Check sheet for the drawn part. Datum: minimum x, y, z corner. Units: mm. A direction names the side the tool comes from. Coordinates: 2 decimals unless noted, no trailing zeros. Order: outer loops, then holes, each group sorted by start corner. A loop starts at its lowest first (then second) coordinate and runs counter-clockwise, first axis right, second up.
Q1. Cross-section at C-C, the plane x = 6. Record the boundary of the cut face in (y, z).
Q2. Cross-section at B-B, the plane z = 5. Record the boundary of the cut face in (x, y), and give its area (3 significant figures).
Q3. Draft check along Z on the marked faces 5, 6, 7 and 8. Enter one of: pulls with the +Z half, pulls with the -Z half, needs draft (parallel to the pull), parting line crosses it, or undercut.
Q4. Thickness scan on line 1 (Y direction, x = 15, z = 45); line 2 (X direction, y = 14, z = 36); line 3 (Z direction, x = 28.5, y = 9.5). Record the ranges inside material, lowest first.
Q5. Set-up check for the marked faces 1, 2, 3 and 4: record each of +Z, -Z, +X, -X, +Y, -Y from which the full face is reachable in a straight line by a thin tool's end or side.
Q6. Depth check by flat-ended pin: P1, Ø1.6, axis at x = 51, y = 1.5, coming from the +Z side; P2, Ø1, axis at x = 47, z = 16.5, coming from the +Y side; P3, Ø1, axis at x = 40.5, y = 1, coming from the -Z side. Enter the tip coordinate at first touch or a pass-through.
Q7. Cross-section at A-A, the plane y = 9.75. Record the boundary of the cut face in (x, z), and give its area (3 significant figures).
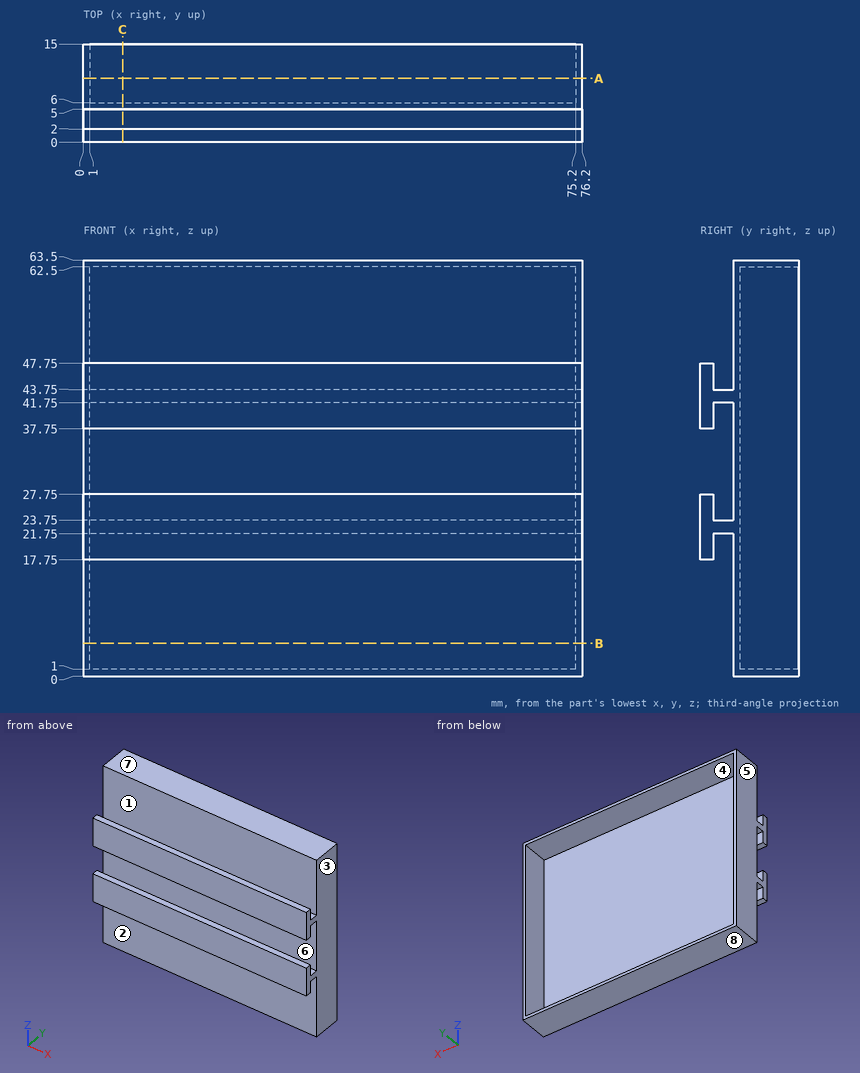
Check values:
1. outline: (0, 17.75) - (2, 17.75) - (2, 21.75) - (5, 21.75) - (5, 0) - (15, 0) - (15, 1) - (6, 1) - (6, 62.5) - (15, 62.5) - (15, 63.5) - (5, 63.5) - (5, 43.75) - (2, 43.75) - (2, 47.75) - (0, 47.75) - (0, 37.75) - (2, 37.75) - (2, 41.75) - (5, 41.75) - (5, 23.75) - (2, 23.75) - (2, 27.75) - (0, 27.75) - close
2. outline: (0, 5) - (76.2, 5) - (76.2, 15) - (75.2, 15) - (75.2, 6) - (1, 6) - (1, 15) - (0, 15) - close
2. area: 94.2 mm2
3. face 5: needs draft
3. face 6: undercut
3. face 7: pulls with the +Z half
3. face 8: pulls with the -Z half
4. line 1: y = 0 to 2, 5 to 6
4. line 2: x = 0 to 1, 75.2 to 76.2
4. line 3: z = 0 to 1, 62.5 to 63.5
5. face 1: +Z, +X, -X
5. face 2: -Z, +X, -X
5. face 3: +Z, -Z, +X, +Y, -Y
5. face 4: +Y
6. P1: stops at z = 47.75
6. P2: stops at y = 6
6. P3: stops at z = 17.75
7. outline: (0, 0) - (76.2, 0) - (76.2, 63.5) - (0, 63.5) - close; hole (1, 1) - (75.2, 1) - (75.2, 62.5) - (1, 62.5) - close
7. area: 275 mm2
